```python
from build123d import *

# Parameters (mm, degrees)
SKETCH1_R           = 5
BOSS_EXTRUDE1_DEPTH = 3
SCALE1_SCALE        = 3


with BuildPart() as part:
    # Sketch1 → Boss-Extrude1 (new body)
    with BuildSketch(Plane.XY):
        with BuildLine():
            ThreePointArc((-41.753986468, 83.099967593), (-43.270314203, 81.314818292), (-43.041341374, 78.983814372))
            Line((-43.041341374, 78.983814372), (-42.998763062, 78.905680247))
            ThreePointArc((-42.998763062, 78.905680247), (-40.153807851, 76.543039354), (-36.463426148, 76.781629011))
            ThreePointArc((-36.463426148, 76.781629011), (0, 85), (36.463426148, 76.781629011))
            ThreePointArc((36.463426148, 76.781629011), (40.153807851, 76.543039354), (42.998763062, 78.905680247))
            Line((42.998763062, 78.905680247), (43.041341374, 78.983814372))
            ThreePointArc((43.041341374, 78.983814372), (43.270314203, 81.314818292), (41.753986468, 83.099967593))
            ThreePointArc((41.753986468, 83.099967593), (41.278907761, 83.336977231), (40.802483763, 83.571270894))
            ThreePointArc((40.802483763, 83.571270894), (39.895257732, 96.043575582), (30.418144359, 87.884791026))
            ThreePointArc((30.418144359, 87.884791026), (0, 93), (-30.418144359, 87.884791026))
            ThreePointArc((-30.418144359, 87.884791026), (-39.895257732, 96.043575582), (-40.802483763, 83.571270894))
            ThreePointArc((-40.802483763, 83.571270894), (-41.278907761, 83.336977231), (-41.753986468, 83.099967593))
        make_face()
        with Locations((-37.21, 89.579104148)):
            Circle(SKETCH1_R, mode=Mode.SUBTRACT)
        with Locations((37.21, 89.579104148)):
            Circle(SKETCH1_R, mode=Mode.SUBTRACT)
    extrude(amount=BOSS_EXTRUDE1_DEPTH)


with BuildPart() as part_1:
    # Scale1: scaled about (0, 86.37118339, 1.5)
    add(part.part.scale(SCALE1_SCALE).moved(Location((0, -172.74236678, -3))))


solid = part_1.part
```
Geometry: final body of the model. Coordinates: model frame, mm. Coordinates: 2 decimals unless noted, no trailing zeros. Write each loop counter-clockwise with the first axis right and the second up, starting at its lowest first coordinate (ties: lowest second). Pieces come first, ordered by that corner, then holes. Notation, with made-up numbers: M -28,29 L -10,29 A14 ccw -10,49 Z; hole C 73.25,-30 d2. An arc over 180 degrees is marked long. Answer as CSV lines item,"result". Start each with the question number.
Q1. Cut plane A-A on x = 111.63. Return the cut outline in (y, z), then the cut area to 3 significant figures.
Q2. Cut plane C-C on x = -51. Return the cut outline in (y, z).
Q3. Cut plane B-B on z = 3. Return the cut outline in (x, y) (3 decimals).
Q4. Line query: line 1 (X direction, y = 90, z = -1.75); line 2 (X direction, y = 89, z = 0); line 3 (Y direction, x = -111.63, z = 1.5). Output: solid intervals per line, ascending. Write a range as from..to.
Q5. Mould query, pull axis Y, two halves, no side actions, for faces 1 (the flat face through (-2, 87, -3)), 2 (the cylindrical face through (120.31, 56.84, 1.44)), 3 (the cylindrical face through (-126.615, 96.654, 1.437)). Classes: released by +Y, released by -Y, zero draft, split by the parting line, or undercut.
Q6. Pin query (flat end, axial travel): P1, Ø1, axis at x = -47, y = 103, coming from the -Z side; P2, Ø5, axis at x = -62.5, z = 1, coming from the +Y side; P3, Ø2, axis at y = 64.5, z = 1, coming from the -X side. Return the tip coordinate at first contact, or that it passes through.
Findings below:
1,outline,"M 56.75,-3 L 80.99,-3 L 80.99,6 L 56.75,6 Z; M 110.99,-3 L 116.99,-3 L 116.99,6 L 110.99,6 Z"
1,area,"272 mm2"
2,outline,"M 77.11,-3 L 101.56,-3 L 101.56,6 L 77.11,6 Z"
3,outline,"M -129.124,64.209 L -128.996,63.975 A15 ccw -109.39,57.603 A255 cw 109.39,57.603 A15 ccw 128.996,63.975 L 129.124,64.209 A9 ccw 125.262,76.558 A279 ccw 122.407,77.971 A21 ccw long 91.254,90.912 A279 ccw -91.254,90.912 A21 ccw long -122.407,77.971 A279 ccw -125.262,76.558 A9 ccw Z; hole C -111.63,95.995 d30; hole C 111.63,95.995 d30"
4,line 1,"x = -131.76..-125.38, -97.88..97.88, 125.38..131.76"
4,line 2,"x = -131.43..-124.9, -98.36..98.36, 124.9..131.43"
4,line 3,"y = 56.75..80.99, 110.99..116.99"
5,face 1,"zero draft"
5,face 2,"released by -Y"
5,face 3,"undercut"
6,P1,"passes through"
6,P2,"stops at y = 99.73"
6,P3,"stops at x = -129.7"
